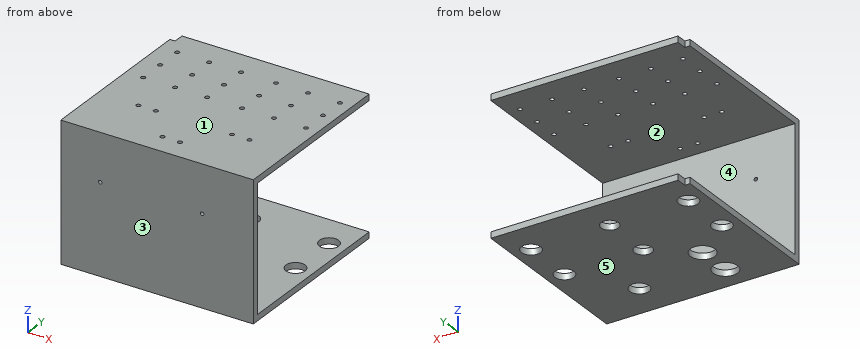
from build123d import *

# Parameters (mm, degrees)
CROQUIS1_W              = 220
CROQUIS1_H              = 204.5
SALIENTE_EXTRUIR1_DEPTH = 7
CROQUIS2_R              = 11
CROQUIS2_R_2            = 10
CROQUIS2_R_3            = 14
CORTAR_EXTRUIR1_DEPTH   = 151.346474851
CROQUIS3_W              = 6
CROQUIS3_H              = 12
CORTAR_EXTRUIR2_DEPTH   = 10
CROQUIS4_W              = 220
CROQUIS4_H              = 7
SALIENTE_EXTRUIR2_DEPTH = 150.6
CROQUIS5_W              = 220
CROQUIS5_H              = 7
SALIENTE_EXTRUIR3_DEPTH = 197.5
CROQUIS6_W              = 6
CROQUIS6_H              = 12
CORTAR_EXTRUIR3_DEPTH   = 150.6
CROQUIS7_R              = 2.5
CORTAR_EXTRUIR4_DEPTH   = 10
CROQUIS8_W              = 20
CROQUIS8_H              = 15
SALIENTE_EXTRUIR4_DEPTH = 197.5
CROQUIS9_W              = 110.5
CROQUIS9_H              = 4
CORTAR_EXTRUIR5_DEPTH   = 94
CROQUIS11_R             = 2.5
CORTAR_EXTRUIR6_DEPTH   = 10
CORTAR_EXTRUIR7_REACH   = 188.514
CROQUIS10_W             = 13.75
CROQUIS10_H             = 75
CORTAR_EXTRUIR8_REACH   = 282.639
CROQUIS12_W             = 10.25034787
CROQUIS12_H             = 5.500172095
CROQUIS12_W_2           = 10.24965213
CROQUIS13_W             = 3
CROQUIS13_H             = 5.499827905
CORTAR_EXTRUIR9_DEPTH   = 7
CORTAR_EXTRUIR10_DEPTH  = 15
SALIENTE_EXTRUIR5_DEPTH = 15
CROQUIS19_R             = 2
CROQUIS19_R_2           = 1.999827905
CORTAR_EXTRUIR13_DEPTH  = 276.579407794
CROQUIS20_W             = 150
CROQUIS20_H             = 15
CORTAR_EXTRUIR14_DEPTH  = 197.5


with BuildPart() as part:
    # Croquis1 → Saliente-Extruir1 (new body)
    with BuildSketch(Plane.XY):
        Rectangle(CROQUIS1_W, CROQUIS1_H)
    extrude(amount=SALIENTE_EXTRUIR1_DEPTH)

    # Croquis2 → Cortar-Extruir1 (cut, through all)
    with BuildSketch(Plane.XY.offset(7)):
        with Locations((-90, 62.25)):
            Circle(CROQUIS2_R)
        with Locations(Location((90, 62.25, 0), (0, 0, 180))):
            Circle(CROQUIS2_R)
        with Locations((0, 62.25)):
            Circle(CROQUIS2_R_2)
        with Locations((90, 3.25)):
            Circle(CROQUIS2_R)
        with Locations(Location((0, 3.25, 0), (0, 0, 180))):
            Circle(CROQUIS2_R_2)
        with Locations(Location((-90, 3.25, 0), (0, 0, 180))):
            Circle(CROQUIS2_R)
        with Locations((-45, -32.25)):
            Circle(CROQUIS2_R_3)
        with Locations((-45, -72.25)):
            Circle(CROQUIS2_R_3)
        with Locations((45, -59.625285127)):
            Circle(CROQUIS2_R)
    extrude(amount=-CORTAR_EXTRUIR1_DEPTH, mode=Mode.SUBTRACT)

    # Croquis3 → Cortar-Extruir2 (cut)
    with BuildSketch(Plane.XY.offset(7)):
        with Locations((-107, 96.25)):
            Rectangle(CROQUIS3_W, CROQUIS3_H)
    extrude(amount=-CORTAR_EXTRUIR2_DEPTH, mode=Mode.SUBTRACT)

    # Croquis4 → Saliente-Extruir2 (add)
    with BuildSketch(Plane.XY.offset(7)):
        with Locations((0, -98.75)):
            Rectangle(CROQUIS4_W, CROQUIS4_H)
    extrude(amount=SALIENTE_EXTRUIR2_DEPTH)

    # Croquis5 → Saliente-Extruir3 (add)
    with BuildSketch(Plane(origin=(0, -95.25, 0), x_dir=(1, 0, 0), z_dir=(0, 1, 0))):
        with Locations((0, -154.1)):
            Rectangle(CROQUIS5_W, CROQUIS5_H)
    extrude(amount=SALIENTE_EXTRUIR3_DEPTH)

    # Croquis6 → Cortar-Extruir3 (cut)
    with BuildSketch(Plane(origin=(0, 0, 150.6), x_dir=(-1, 0, 0), z_dir=(0, 0, -1))):
        with Locations((107, 96.25)):
            Rectangle(CROQUIS6_W, CROQUIS6_H)
    extrude(amount=-CORTAR_EXTRUIR3_DEPTH, mode=Mode.SUBTRACT)

    # Croquis7 → Cortar-Extruir4 (cut)
    with BuildSketch(Plane.XY.offset(157.6)):
        with Locations((-90, 72.25)):
            Circle(CROQUIS7_R)
        with Locations((-17, 72.25)):
            Circle(CROQUIS7_R)
        with Locations((-53.5, 72.25)):
            Circle(CROQUIS7_R)
        with Locations((96, 72.25)):
            Circle(CROQUIS7_R)
        with Locations((59.5, 72.25)):
            Circle(CROQUIS7_R)
        with Locations((23, 72.25)):
            Circle(CROQUIS7_R)
        with Locations((96, 42.25)):
            Circle(CROQUIS7_R)
        with Locations((59.5, 42.25)):
            Circle(CROQUIS7_R)
        with Locations((23, 42.25)):
            Circle(CROQUIS7_R)
        with Locations((-17, 42.25)):
            Circle(CROQUIS7_R)
        with Locations((-53.5, 42.25)):
            Circle(CROQUIS7_R)
        with Locations((-90, 42.25)):
            Circle(CROQUIS7_R)
        with Locations((96, 12.25)):
            Circle(CROQUIS7_R)
        with Locations((59.5, 12.25)):
            Circle(CROQUIS7_R)
        with Locations((23, 12.25)):
            Circle(CROQUIS7_R)
        with Locations((-17, 12.25)):
            Circle(CROQUIS7_R)
        with Locations((-53.5, 12.25)):
            Circle(CROQUIS7_R)
        with Locations((-90, 12.25)):
            Circle(CROQUIS7_R)
    extrude(amount=-CORTAR_EXTRUIR4_DEPTH, mode=Mode.SUBTRACT)

    # Croquis8 → Saliente-Extruir4 (add)
    with BuildSketch(Plane(origin=(0, -95.25, 0), x_dir=(1, 0, 0), z_dir=(0, 1, 0))):
        with Locations((-50, -103.1)):
            Rectangle(CROQUIS8_W, CROQUIS8_H)
        with Locations((50, -103.1)):
            Rectangle(CROQUIS8_W, CROQUIS8_H)
    extrude(amount=SALIENTE_EXTRUIR4_DEPTH)

    # Croquis9 → Cortar-Extruir5 (cut)
    with BuildSketch(Plane(origin=(0, 102.25, 0), x_dir=(1, 0, 0), z_dir=(0, 1, 0))):
        with Locations((-0.00034787, -103.099827905)):
            Rectangle(CROQUIS9_W, CROQUIS9_H)
    extrude(amount=-CORTAR_EXTRUIR5_DEPTH, mode=Mode.SUBTRACT)

    # Croquis11 → Cortar-Extruir6 (cut)
    with BuildSketch(Plane.XY.offset(157.6)):
        with Locations((-10, -77.25)):
            Circle(CROQUIS11_R)
        with Locations((10, -77.25)):
            Circle(CROQUIS11_R)
        with Locations((-63.5, -37.25)):
            Circle(CROQUIS11_R)
        with Locations((-43.5, -37.25)):
            Circle(CROQUIS11_R)
        with Locations((43.5, -37.25)):
            Circle(CROQUIS11_R)
        with Locations((63.5, -37.25)):
            Circle(CROQUIS11_R)
    extrude(amount=-CORTAR_EXTRUIR6_DEPTH, mode=Mode.SUBTRACT)

    # Cortar-Extruir7: up to this face of the body (flat: up to its plane)
    cortar_extruir7_end = Plane(part.part.faces().sort_by_distance((-50, 3.5, 95.6))[0])
    # Croquis10 → Cortar-Extruir7 (cut, up to the picked face)
    with BuildSketch(Plane.XY.offset(110.6), mode=Mode.PRIVATE) as cortar_extruir7_sk1:
        with Locations((-46.875, 57.75)):
            Rectangle(CROQUIS10_W, CROQUIS10_H)
    cortar_extruir7_tool1 = split(extrude(cortar_extruir7_sk1.sketch, amount=-CORTAR_EXTRUIR7_REACH, mode=Mode.PRIVATE), bisect_by=cortar_extruir7_end, keep=Keep.BOTH, mode=Mode.PRIVATE)
    # Croquis10 → Cortar-Extruir7 (cut, up to the picked face)
    with BuildSketch(Plane.XY.offset(110.6), mode=Mode.PRIVATE) as cortar_extruir7_sk2:
        with Locations((46.875, 57.75)):
            Rectangle(CROQUIS10_W, CROQUIS10_H)
    cortar_extruir7_tool2 = split(extrude(cortar_extruir7_sk2.sketch, amount=-CORTAR_EXTRUIR7_REACH, mode=Mode.PRIVATE), bisect_by=cortar_extruir7_end, keep=Keep.BOTH, mode=Mode.PRIVATE)
    add(cortar_extruir7_tool1.solids().sort_by(Axis((-46.875, 57.75, 110.6), (0, 0, -1)))[0], mode=Mode.SUBTRACT)
    add(cortar_extruir7_tool2.solids().sort_by(Axis((46.875, 57.75, 110.6), (0, 0, -1)))[0], mode=Mode.SUBTRACT)

    # Cortar-Extruir8: up to this face of the body (flat: up to its plane)
    cortar_extruir8_end = Plane(part.part.faces().sort_by_distance((-47.625173935, 8.25, 103.099827905))[0])
    # Croquis12 → Cortar-Extruir8 (cut, up to the picked face)
    with BuildSketch(Plane(origin=(0, 102.25, 0), x_dir=(1, 0, 0), z_dir=(0, 1, 0)), mode=Mode.PRIVATE) as cortar_extruir8_sk1:
        with Locations((-45.125173935, -107.849913953)):
            Rectangle(CROQUIS12_W, CROQUIS12_H)
    cortar_extruir8_tool1 = split(extrude(cortar_extruir8_sk1.sketch, amount=-CORTAR_EXTRUIR8_REACH, mode=Mode.PRIVATE), bisect_by=cortar_extruir8_end, keep=Keep.BOTH, mode=Mode.PRIVATE)
    # Croquis12 → Cortar-Extruir8 (cut, up to the picked face)
    with BuildSketch(Plane(origin=(0, 102.25, 0), x_dir=(1, 0, 0), z_dir=(0, 1, 0)), mode=Mode.PRIVATE) as cortar_extruir8_sk2:
        with Locations((45.124826065, -107.849913953)):
            Rectangle(CROQUIS12_W_2, CROQUIS12_H)
    cortar_extruir8_tool2 = split(extrude(cortar_extruir8_sk2.sketch, amount=-CORTAR_EXTRUIR8_REACH, mode=Mode.PRIVATE), bisect_by=cortar_extruir8_end, keep=Keep.BOTH, mode=Mode.PRIVATE)
    add(cortar_extruir8_tool1.solids().sort_by(Axis((-45.125174, 102.25, 107.849914), (0, -1, 0)))[0], mode=Mode.SUBTRACT)
    add(cortar_extruir8_tool2.solids().sort_by(Axis((45.124826, 102.25, 107.849914), (0, -1, 0)))[0], mode=Mode.SUBTRACT)

    # Croquis13 → Cortar-Extruir9 (cut)
    with BuildSketch(Plane(origin=(0, 102.25, 0), x_dir=(1, 0, 0), z_dir=(0, 1, 0))):
        with Locations((-41.5, -98.349913953)):
            Rectangle(CROQUIS13_W, CROQUIS13_H)
        with Locations((41.5, -98.349913953)):
            Rectangle(CROQUIS13_W, CROQUIS13_H)
    extrude(amount=-CORTAR_EXTRUIR9_DEPTH, mode=Mode.SUBTRACT)

    # Croquis14 → Cortar-Extruir10 (cut)
    with BuildSketch(Plane.XY.offset(110.6)):
        Polygon((-40, -10.25), (-51.479605867, -10.25), (-60, -10.25), (-60, -60.25), (-40, -60.25), align=None)
    extrude(amount=-CORTAR_EXTRUIR10_DEPTH, mode=Mode.SUBTRACT)


with BuildPart() as cortar_extruir10_piece_1:
    # of the separate pieces the step leaves, piece 1, a body of its own (cortar_extruir10_pieces)
    add(part.part.solids().sort_by_distance((-104, 102.25, 0))[0])



with BuildPart() as cortar_extruir10_piece_2:
    # of the separate pieces the step leaves, piece 2, a body of its own (cortar_extruir10_pieces)
    add(part.part.solids().sort_by_distance((-40, -10.25, 95.6))[0])


with BuildPart() as cortar_extruir10_piece_1_1:
    add(cortar_extruir10_piece_1.part)

    add(cortar_extruir10_piece_2.part)  # Saliente-Extruir5 merges Cortar-Extruir10 piece 2
    # Croquis15 → Saliente-Extruir5 (add)
    with BuildSketch(Plane.XY.offset(110.6)):
        Polygon((-60, 19.75), (-90, 19.75), (-90, -95.25), (-60, -95.25), (-60, -60.25), (-66.476045764, -60.25), (-66.476045764, -10.25), (-60, -10.25), align=None)
    extrude(amount=-SALIENTE_EXTRUIR5_DEPTH)

    # Croquis19 → Cortar-Extruir13 (cut, through all)
    with BuildSketch(Plane(origin=(0, -95.25, 0), x_dir=(1, 0, 0), z_dir=(0, 1, 0))):
        with Locations(Location((-65, -103.1, 0), (0, 0, 270))):
            Circle(CROQUIS19_R)
        with Locations(Location((51.5, -103.1, 0), (0, 0, 270))):
            Circle(CROQUIS19_R_2)
    extrude(amount=-CORTAR_EXTRUIR13_DEPTH, mode=Mode.SUBTRACT)

    # Croquis20 → Cortar-Extruir14 (cut)
    with BuildSketch(Plane(origin=(0, 102.25, 0), x_dir=(1, 0, 0), z_dir=(0, 1, 0))):
        with Locations((-15, -103.1)):
            Rectangle(CROQUIS20_W, CROQUIS20_H)
    extrude(amount=-CORTAR_EXTRUIR14_DEPTH, mode=Mode.SUBTRACT)


solid = cortar_extruir10_piece_1_1.part
Design review of the part built by this model. Coordinates are the model's own, in mm. Face numbers are marked on the shaded views. A direction names the side the tool comes from. Round coordinates to 2 decimals unless told otherwise and drop trailing zeros. Write each loop counter-clockwise with the first axis right and the second up, starting at its lowest first coordinate (ties: lowest second). Pieces come first, ordered by that corner, then holes. Notation, with made-up numbers: (-35.5, 39.25) -> (2.5, 39.25) arc R13 cw to (2.5, 46.25) -> close; hole circle Ø11 at (47.5, 14.25). An arc over 180 degrees is marked (long way). One line per question, with ' | ' between items.
(1) Take a section at D-D, the plane x = 0.5. State the section outline as (y, z) points.
Result sheet:
outline: (-102.25, 0) -> (-6.74, 0) -> (-6.74, 7) -> (-95.25, 7) -> (-95.25, 150.6) -> (102.25, 150.6) -> (102.25, 157.6) -> (-102.25, 157.6) -> close; (13.24, 0) -> (52.26, 0) -> (52.26, 7) -> (13.24, 7) -> close; (72.24, 0) -> (102.25, 0) -> (102.25, 7) -> (72.24, 7) -> close
(2) Machinability: for the marked faces 1 and 2, which of the approach directions +Z, -Z, +X, -X, +Y, -Y give a long, thin tool a straight path to every point of the face, cutting with its end or side? Answer none if there is none.
Result sheet:
face 1: +Z, +X, -X, +Y, -Y | face 2: +X, -X, +Y
(3) Take a section at B-B, the plane x = 90. State the section outline as (y, z) points, and give its area (3 significant figures).
Result sheet:
outline: (-102.25, 0) -> (-7.75, 0) -> (-7.75, 7) -> (-95.25, 7) -> (-95.25, 150.6) -> (102.25, 150.6) -> (102.25, 157.6) -> (-102.25, 157.6) -> close; (14.25, 0) -> (51.25, 0) -> (51.25, 7) -> (14.25, 7) -> close; (73.25, 0) -> (102.25, 0) -> (102.25, 7) -> (73.25, 7) -> close | area: 3,560 mm2
(4) Draft analysis for pull direction Z (two halves, no side actions). For the marked faces 3, 4 and 5, state which applies: released by +Z, released by -Z, zero draft, split by the parting line, or undercut.
Result sheet:
face 3: zero draft | face 4: undercut | face 5: released by -Z
(5) Insertion check: P1, Ø5, axis at x = 33.5, z = 111.5, coming from the +Y side; P2, Ø5.5, axis at y = 96.5, z = 153, coming from the -X side. Each pin has a flat end and moves straight along its axis. Give the tip position at first contact, or say it passes through.
Result sheet:
P1: y = -95.25 | P2: x = -104
(6) Take a section at C-C, the plane z = 86.5. State the section outline as (x, y) points.
Result sheet:
outline: (-110, -102.25) -> (110, -102.25) -> (110, -95.25) -> (-110, -95.25) -> close
(7) Wall thickness on line 1 (Z direction, x = 23, y = -65); line 2 (Y direction, x = 0, z = 2); line 3 (Y direction, x = 63.5, z = 154.5): over which ranges is each line inside the solid? List them lowest first. Write a range as [from, to].
Result sheet:
line 1: [0, 7], [150.6, 157.6] | line 2: [-102.25, -6.75], [13.25, 52.25], [72.25, 102.25] | line 3: [-102.25, -39.75], [-34.75, 102.25]
(8) Take a section at A-A, the plane y = 81.5. State the section outline as (x, z) points.
Result sheet:
outline: (-110, 0) -> (110, 0) -> (110, 7) -> (-110, 7) -> close; (-110, 150.6) -> (110, 150.6) -> (110, 157.6) -> (-110, 157.6) -> close
